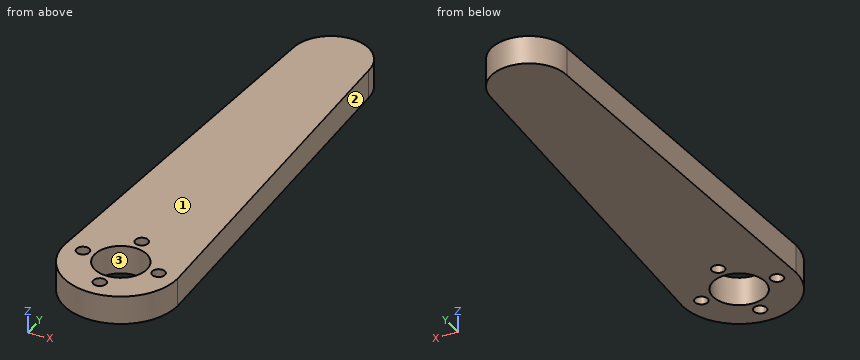
from build123d import *

# Parameters (mm, degrees)
BOSS_EXTRU_1_DEPTH           = 6
ESQUISSE2_R                  = 5.5
ESQUISSE2_R_2                = 1.35
ENL_V_MAT_EXTRU_1_DEPTH      = 1
ENL_V_MAT_EXTRU_1_DEPTH_BACK = 7


with BuildPart() as part:
    # Esquisse1 → Boss.-Extru.1 (new body)
    with BuildSketch(Plane.XY):
        with BuildLine():
            Line((12, 0), (8, 80))
            ThreePointArc((8, 80), (0, 88), (-8, 80))
            Line((-8, 80), (-12, 0))
            ThreePointArc((-12, 0), (0, -12), (12, 0))
        make_face()
    extrude(amount=BOSS_EXTRU_1_DEPTH)

    # Esquisse2 → Enlèv. mat.-Extru.1 (cut, two sides)
    with BuildSketch(Plane.XY.offset(6)) as enl_v_mat_extru_1_sk:
        Circle(ESQUISSE2_R)
        with Locations((8, 0)):
            Circle(ESQUISSE2_R_2)
        with Locations((0, -8)):
            Circle(ESQUISSE2_R_2)
        with Locations((-8, 0)):
            Circle(ESQUISSE2_R_2)
        with Locations((0, 8)):
            Circle(ESQUISSE2_R_2)
    extrude(amount=ENL_V_MAT_EXTRU_1_DEPTH, mode=Mode.SUBTRACT)
    extrude(enl_v_mat_extru_1_sk.sketch, amount=-ENL_V_MAT_EXTRU_1_DEPTH_BACK, mode=Mode.SUBTRACT)


solid = part.part
Source: CAD feature listing. Evaluate the final solid. Frame: model axes, mm. Face numbers are marked on the shaded views. Round coordinates to 2 decimals unless told otherwise and drop trailing zeros. Loops run counter-clockwise (first coordinate to the right, second up) from the corner with the lowest first, then second, coordinate; pieces in that order, holes last.
Q1. Section D-D, the plane y = -8. Return loops of the section in (x, z), plus the area to 3 significant figures.
Q2. Ray query, line 1 (Y direction, x = 0, z = 4.15); line 2 (X direction, y = 7, z = 0.65); line 3 (X direction, y = 6.5, z = 2.95) (3 decimals). Return the intervals inside material, ascending.
Q3. Mould query, pull axis Y, two halves, no side actions, for the marked faces 1, 2 and 3. Classes: pulls with the +Y half, pulls with the -Y half, needs draft (parallel to the pull), parting line crosses it, or undercut.
Q4. Section A-A, the plane y = 8. Return loops of the section in (x, z).
Q5. Section B-B, the plane z = 2.6. Return loops of the section in (x, y), plus the area to 3 significant figures.
Q6. First-contact query: P1, Ø2.5, axis at x = 0, y = 8, coming from the +Z side. Flat tip, straight axial feed; report the tip coordinate or a pass-through.
Q7. Section C-C, the plane x = 0. Return loops of the section in (y, z).
Solutions:
1. outline: (-8.94, 0) - (-1.35, 0) - (-1.35, 6) - (-8.94, 6) - close; (1.35, 0) - (8.94, 0) - (8.94, 6) - (1.35, 6) - close
1. area: 91.1 mm2
2. line 1: y = -12 to -9.35, -6.65 to -5.5, 5.5 to 6.65, 9.35 to 88
2. line 2: x = -11.65 to -0.91, 0.91 to 11.65
2. line 3: x = -11.675 to 11.675
3. face 1: needs draft
3. face 2: pulls with the +Y half
3. face 3: undercut
4. outline: (-11.6, 0) - (-1.35, 0) - (-1.35, 6) - (-11.6, 6) - close; (1.35, 0) - (11.6, 0) - (11.6, 6) - (1.35, 6) - close
5. outline: (-12, 0) arc R12 ccw to (12, 0) - (8, 80) arc R8 ccw to (-8, 80) - close; hole circle Ø2.7 at (-8, 0); hole circle Ø11 at (0, 0); hole circle Ø2.7 at (0, -8); hole circle Ø2.7 at (0, 8); hole circle Ø2.7 at (8, 0)
5. area: 1,810 mm2
6. P1: passes through
7. outline: (-12, 0) - (-9.35, 0) - (-9.35, 6) - (-12, 6) - close; (-6.65, 0) - (-5.5, 0) - (-5.5, 6) - (-6.65, 6) - close; (5.5, 0) - (6.65, 0) - (6.65, 6) - (5.5, 6) - close; (9.35, 0) - (88, 0) - (88, 6) - (9.35, 6) - close
